Model file for the job. Use its own axes, mm. A direction names the side the tool comes from. Coordinates: 2 decimals unless noted, no trailing zeros. Write each loop counter-clockwise with the first axis right and the second up, starting at its lowest first coordinate (ties: lowest second). Pieces come first, ordered by that corner, then holes.
Q1. Band-saw the part on A-A, the plane x = 0. Write the cut outline in (y, z), plus the area to 3 significant figures.
Q2. Band-saw the part on C-C, the plane z = 88.5. Write the cut outline in (x, y).
Q3. Which spindle directions (+Z, -Z, +X, -X, +Y, -Y) get a long thin tool onto all of the face, cutting with end or side? Do faces 1 (the cylindrical face through (-16.18, -72.86, 150.93)), 2 (the flat face through (75, -1, 8)), 3 (the flat face through (32, 51, 16)). Say none if no direction does.
Q4. Drill centre lines: probe 1 along Y at (x, z) = (0, 153); probe 2 along Z at (x, y) = (-67.5, 27.5); probe 3 along Y at (x, z) = (0, 58). Where is each one in solid material? Low to high.
Q5. Pin check, flat tips, straight feed: P1, Ø3, axis at y = 42, z = 91, coming from the -X side; P2, Ø1, axis at x = -42.5, z = 93, coming from the +Y side; P3, Ø3, axis at y = -28, z = 78.5, coming from the +X side. Stop position of each tip, or through.
Q6. Band-saw the part on D-D, the plane x = 54. Write the cut outline in (y, z).
Q7. Pull direction Z, two halves, no side cores. Call faces 4 (the flat face through (38, -44, 146)), 5 (the flat face through (-1, -75, 8)), 6 (the flat face through (-1, 51, 0)): released by +Z, released by -Z, zero draft, split by the parting line, or undercut.
from build123d import *

# Parameters (mm, degrees)
F0_W      = 150
F0_H      = 150
F1_DEPTH  = 16
F2_R      = 3.2
F4_R      = 57.5
F5_DEPTH  = 130
F6_R      = 50
F7_DEPTH  = 146.001
F9_R      = 74.633597
F9_R_2    = 50
F10_DEPTH = 10


with BuildPart() as f1:
    # F0 (on Top) → F1 (new body)
    with BuildSketch(Plane.XY):
        Rectangle(F0_W, F0_H)
    extrude(amount=F1_DEPTH)

    # F2
    f2_edges = [f1.edges().sort_by_distance(p)[0] for p in [
        (-75, 75, 8),
        (75, 75, 8),
        (75, -75, 8),
        (-75, -75, 8),
    ]]
    fillet(f2_edges, radius=F2_R)

    # F4 (on face) → F5 (join)
    with BuildSketch(Plane.XY.offset(16)):
        Circle(F4_R)
    extrude(amount=F5_DEPTH)

    # F6 (on face) → F7 (cut, through all)
    with BuildSketch(Plane.XY.offset(146)):
        Circle(F6_R)
    extrude(amount=-F7_DEPTH, mode=Mode.SUBTRACT)

    # F9 (on face) → F10 (join)
    with BuildSketch(Plane.XY.offset(146)):
        Circle(F9_R)
        Circle(F9_R_2, mode=Mode.SUBTRACT)
    extrude(amount=F10_DEPTH)


solid = f1.part
Answer sheet:
1. outline: (-75, 0) - (-50, 0) - (-50, 156) - (-74.63, 156) - (-74.63, 146) - (-57.5, 146) - (-57.5, 16) - (-75, 16) - close; (50, 0) - (75, 0) - (75, 16) - (57.5, 16) - (57.5, 146) - (74.63, 146) - (74.63, 156) - (50, 156) - close
1. area: 3,240 mm2
2. outline: circle Ø115 at (0, 0); hole circle Ø100 at (0, 0)
3. face 1: +Z
3. face 2: +Z, -Z, +X, +Y, -Y
3. face 3: none
4. probe 1: y = -74.63 to -50, 50 to 74.63
4. probe 2: z = 0 to 16, 146 to 156
4. probe 3: y = -57.5 to -50, 50 to 57.5
5. P1: stops at x = -40.82
5. P2: stops at y = 39.27
5. P3: stops at x = 51.03
6. outline: (-75, 0) - (75, 0) - (75, 16) - (19.75, 16) - (19.75, 146) - (51.52, 146) - (51.52, 156) - (-51.52, 156) - (-51.52, 146) - (-19.75, 146) - (-19.75, 16) - (-75, 16) - close
7. face 4: undercut
7. face 5: zero draft
7. face 6: released by -Z
